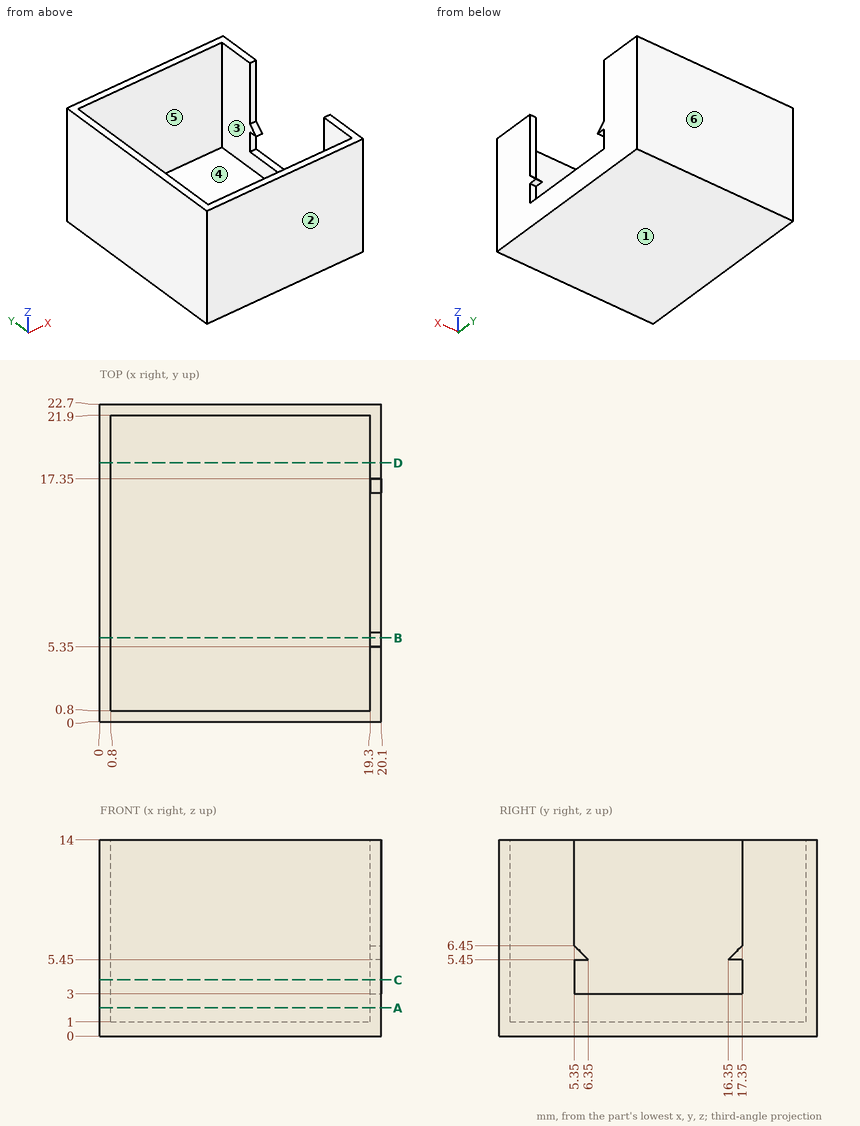
Source: three-view drawing plus pictorial views. Frame: mm from the lowest corner of the part. A direction names the side the tool comes from. Give positions to 0.01 mm unless a question says otherwise; leave off trailing zeros. Write each loop counter-clockwise with the first axis right and the second up, starting at its lowest first coordinate (ties: lowest second). Pieces come first, ordered by that corner, then holes.
(1) Cut plane C-C, the plane z = 4. Return loops of the section in (x, y), then the cut area to 3 significant figures.
(2) First-contact query: P1, Ø8, axis at x = 11, y = 14, coming from the +Z side. Flat tip, straight axial feed; report the tip coordinate or a pass-through.
(3) Cut plane D-D, the plane y = 18.5. Return loops of the section in (x, z), then the cut area to 3 significant figures.
(4) Access query for the marked faces 5 and 6. Directions: +Z, -Z, +X, -X, +Y, -Y. A direction counts if a zero-diameter tool reaches every point of the face in a straight line with its end or side. Return the directions, or none.
(5) Cut plane A-A, the plane z = 2. Return loops of the section in (x, y), then the cut area to 3 significant figures.
(6) Ray query, line 1 (X direction, y = 21, z = 3.75); line 2 (Y direction, x = 17, z = 10.5); line 3 (X direction, y = 16.75, z = 11). Return the intervals inside material, ascending.
(7) Cut plane B-B, the plane y = 6. Return loops of the section in (x, z), then the cut area to 3 significant figures.
(8) Mould query, pull axis Y, two halves, no side actions, for the marked faces 1, 2, 3 and 4. Classes: released by +Y, released by -Y, zero draft, split by the parting line, or undercut.
Values follow:
1. outline: (0, 0) - (20.1, 0) - (20.1, 5.35) - (19.3, 5.35) - (19.3, 0.8) - (0.8, 0.8) - (0.8, 21.9) - (19.3, 21.9) - (19.3, 17.35) - (20.1, 17.35) - (20.1, 22.7) - (0, 22.7) - close
1. area: 56.3 mm2
2. P1: stops at z = 1
3. outline: (0, 0) - (20.1, 0) - (20.1, 14) - (19.3, 14) - (19.3, 1) - (0.8, 1) - (0.8, 14) - (0, 14) - close
3. area: 40.9 mm2
4. face 5: +Z
4. face 6: +Z, -Z, +X, -X, +Y
5. outline: (0, 0) - (20.1, 0) - (20.1, 22.7) - (0, 22.7) - close; hole (0.8, 0.8) - (19.3, 0.8) - (19.3, 21.9) - (0.8, 21.9) - close
5. area: 65.9 mm2
6. line 1: x = 0 to 0.8, 19.3 to 20.1
6. line 2: y = 0 to 0.8, 21.9 to 22.7
6. line 3: x = 0 to 0.8
7. outline: (0, 0) - (20.1, 0) - (20.1, 3) - (19.3, 3) - (19.3, 1) - (0.8, 1) - (0.8, 14) - (0, 14) - close; (19.3, 5.45) - (20.1, 5.45) - (20.1, 5.8) - (19.3, 5.8) - close
7. area: 32.4 mm2
8. face 1: zero draft
8. face 2: released by -Y
8. face 3: undercut
8. face 4: undercut
